from build123d import *

# Parameters (mm, degrees)
F0_W     = 25
F0_H     = 25
F0_W_2   = 24
F0_H_2   = 24
F1_DEPTH = 435
F3_DEPTH = 25.001


with BuildPart() as f1:
    # F0 (on Top) → F1 (new body)
    with BuildSketch(Plane.XY):
        with Locations((12.5, -12.5)):
            Rectangle(F0_W, F0_H)
        with Locations((12.5, -12.5)):
            Rectangle(F0_W_2, F0_H_2, mode=Mode.SUBTRACT)
    extrude(amount=F1_DEPTH)

    # F2 (on face) → F3 (cut, through all)
    with BuildSketch(Plane.XZ.offset(25)):
        with BuildLine():
            ThreePointArc((12.348425, 230.002893), (15.773518, 231.525113), (17.17836, 235))
            ThreePointArc((17.17836, 235), (15.776087, 238.472228), (12.355814, 239.99685))
            Line((12.355814, 239.99685), (12.348425, 230.002893))
        make_face()
        with BuildLine():
            Line((12.348425, 230.002893), (12.355814, 239.99685))
            ThreePointArc((12.355814, 239.99685), (7.178362, 235.003697), (12.348425, 230.002893))
        make_face()
    extrude(amount=-F3_DEPTH, mode=Mode.SUBTRACT)


solid = f1.part
The model under review builds one solid part; all positions refer to its coordinate system, in mm. A direction names the side the tool comes from. Give positions to 0.01 mm unless a question says otherwise; leave off trailing zeros. Loops run counter-clockwise (first coordinate to the right, second up) from the corner with the lowest first, then second, coordinate; pieces in that order, holes last. Notation, with made-up numbers: (75, -10) -> (92, -10) arc R24 cw to (92, 14) -> close; hole circle Ø10 at (-29, 78). An arc over 180 degrees is marked (long way). Put each result on its own line as item: value. Start each with the question number.
1. We need section B-B on z = 174. State the section outline as (x, y) points.
2. We need section A-A on y = -16.75. State the section outline as (x, z) points, then the cut area to 3 significant figures.
3. Wall thickness on probe 1 along X at (y, z) = (-23.25, 382); probe 2 along Y at (x, z) = (16, 303): over which ranges is each line inside the solid? List them lowest first.
4. For faces 4 (the face through (0.5, -13, 214)), 5 (the face through (12, -25, 214)), list the 3-axis set-ups (+Z, -Z, +X, -X, +Y, -Y) from which the entire face can be reached by the end or side of a thin tool; tool diameter is ignored.
5. Mouldability with a two-part tool opening along Y and no side actions: class faces 1 (the face through (0, -13, 214)), 2 (the face through (12, -0.5, 214)), 3 (the face through (12, 0, 214)) as released by +Y, released by -Y, zero draft, split by the parting line, or undercut.
Determined:
1. outline: (0, -25) -> (25, -25) -> (25, 0) -> (0, 0) -> close; hole (0.5, -24.5) -> (24.5, -24.5) -> (24.5, -0.5) -> (0.5, -0.5) -> close
2. outline: (0, 0) -> (0.5, 0) -> (0.5, 435) -> (0, 435) -> close; (24.5, 0) -> (25, 0) -> (25, 435) -> (24.5, 435) -> close
2. area: 435 mm^2
3. probe 1: 0 to 0.5, 24.5 to 25
3. probe 2: -25 to -24.5, -0.5 to 0
4. face 4: +Z, -Z
4. face 5: +Z, -Z, +X, -X, -Y
5. face 1: zero draft
5. face 2: undercut
5. face 3: released by +Y
